Read the model definition and answer for the solid it produces. Units are mm, in the model's axes. A direction names the side the tool comes from. Give positions to 0.01 mm unless a question says otherwise; leave off trailing zeros. Order: outer loops, then holes, each group sorted by start corner. A loop starts at its lowest first (then second) coordinate and runs counter-clockwise, first axis right, second up.
Item 1: A cutting plane is placed at A-A (y = 0). Write down the section's boundary in (x, z).
Item 2: Which of the six approach directions +Z, -Z, +X, -X, +Y, -Y give full straight-line access (tool end or side, diameter ignored) to faces 4 (the face through (66, 1, -6.713)), 5 (the face through (36.49, -0.38, 2.48))?
Item 3: The mould has two halves that part along Z. Classify faces 1 (the face through (71, 0, 0)), 2 (the face through (68.597, 1.993, -2.272)), 3 (the face through (0.705, 2.797, 0.101)): +Z half, -Z half, draft (parallel to the pull), parting line (faces both ways), or undercut.
Item 4: A cutting plane is placed at B-B (x = 3). Write down the section's boundary in (y, z).
Item 5: Given pin 1 Ø4 at (x, y) = (37, -0.5) entering from -Z; pin 2 Ø4 at (y, z) = (1, 0.5) entering from -X; pin 3 Ø3 at (x, z) = (52.5, -2) entering from -Y; pin 4 Ø2 at (x, z) = (8.5, -4) entering from -Y, each flat-ended and moving along its own axis, determine where each tip first touches the part or whether it passes through.
Item 6: A cutting plane is placed at C-C (y = 5.5). Write down the section's boundary in (x, z).
Item 7: Find the intervals of material crossed by line 1 along X through (y, z) = (-1, -0.25); line 2 along Z through (x, y) = (18, -1); line 3 along X through (y, z) = (0.5, -6), in increasing order.
Item 8: A cutting plane is placed at D-D (x = 25). Write down the section's boundary in (y, z).
from build123d import *

# Parameters (mm, degrees)
F3_R     = 2.5
F4_DEPTH = 35


with BuildPart() as f1:
    # F0 (on Top) → F1 (revolve)
    with BuildSketch(Plane.XY):
        with BuildLine():
            Line((3, 10.3863353059), (3, 7.9742954113))
            Line((3, 7.9742954113), (5.297709696, 7.9742954113))
            Line((5.297709696, 7.9742954113), (5.297709696, 10.7682199602))
            Line((5.297709696, 10.7682199602), (5.297709696, 11.2461591464))
            ThreePointArc((5.297709696, 11.2461591464), (4.226658763, 10.6083316025), (3, 10.3863353059))
        make_face()
        with BuildLine():
            Line((3, 11.1363353059), (3, 10.3863353059))
            ThreePointArc((3, 10.3863353059), (4.226658763, 10.6083316025), (5.297709696, 11.2461591464))
            ThreePointArc((5.297709696, 11.2461591464), (6.3937863673, 13.0306402124), (6.2748163897, 15.1214780561))
            Line((6.2748163897, 15.1214780561), (5.4570149341, 15.1214780561))
            ThreePointArc((5.4570149341, 15.1214780561), (5.3408484106, 12.4430998024), (3, 11.1363353059))
        make_face()
    revolve(axis=Axis((3, 12.1363353059, 0), (0, -1, 0)))

    # F3 (on offset) → F4 (join, symmetric)
    with BuildSketch(Plane.YZ.offset(36)):
        with Locations((7.1499980986, 0)):
            Circle(F3_R)
    extrude(amount=F4_DEPTH, both=True)


with BuildPart() as f1_1:
    # F5: moved
    add(f1.part.moved(Location((0, -7.2, 0))))

    # F6 (on Front) → F7 (revolve)
    with BuildSketch(Plane.XZ):
        with BuildLine():
            ThreePointArc((68.8586309552, -2.7275545988), (71.1994793659, -4.0343190953), (71.3156458893, -6.712697349))
            Line((71.3156458893, -6.712697349), (72.133447345, -6.712697349))
            ThreePointArc((72.133447345, -6.712697349), (72.2031454778, -4.4459429431), (70.8686844446, -2.612299816))
            ThreePointArc((70.8686844446, -2.612299816), (69.9125778847, -2.1400112103), (68.8586309552, -1.9775545988))
            Line((68.8586309552, -1.9775545988), (68.8586309552, -2.7275545988))
        make_face()
        with BuildLine():
            Line((68.8586309552, 0.4344852958), (68.8586309552, -1.9775545988))
            ThreePointArc((68.8586309552, -1.9775545988), (69.9125778847, -2.1400112103), (70.8686844446, -2.612299816))
            Line((70.8686844446, -2.612299816), (70.8686844446, 0.4344852958))
            Line((70.8686844446, 0.4344852958), (68.8586309552, 0.4344852958))
        make_face()
    revolve(axis=Axis((68.8586309552, 0, -3.7275545988), (0, 0, 1)))


solid = f1_1.part
Response values:
1. outline: (1, -2.5) - (66.85, -2.5) - (66.85, -2.61) arc R3.5 ccw to (65.58, -6.71) - (66.4, -6.71) arc R2.75 cw (long way) to (71.32, -6.71) - (72.13, -6.71) arc R3.5 ccw to (70.87, -2.61) - (70.87, -2.5) - (71, -2.5) - (71, 2.5) - (1, 2.5) - close
2. face 4: -Z, +X, -X, +Y, -Y
2. face 5: none
3. face 1: draft
3. face 2: undercut
3. face 3: parting line
4. outline: (0.94, -2.3) - (4.05, -2.3) arc R3.5 ccw to (7.92, -3.27) - (7.92, -2.46) arc R2.75 cw (long way) to (7.92, 2.46) - (7.92, 3.27) arc R3.5 ccw to (4.05, 2.3) - (0.94, 2.3) arc R2.5 ccw (long way) to start
5. pin 1: stops at z = -2.5
5. pin 2: stops at x = 0.7
5. pin 3: stops at y = -2.5
5. pin 4: passes through
6. outline: circle Ø6.59 at (3, 0); hole circle Ø4.96 at (3, 0)
7. line 1: x = 1 to 71
7. line 2: z = -2.31 to 2.31
7. line 3: x = 65.43 to 66.21, 71.51 to 72.28
8. outline: circle Ø5 at (-0.05, 0)
